Here's the drawing with two shaded views (mm, measured from the low corner). I have some questions. Round coordinates to 2 decimals unless told otherwise and drop trailing zeros. Order: outer loops, then holes, each group sorted by start corner. A loop starts at its lowest first (then second) coordinate and runs counter-clockwise, first axis right, second up. Notation, with made-up numbers: (46, 14) -> (54, 14) arc R22 cw to (54, 42) -> close; hole circle Ø2 at (18.5, 48.25). An arc over 180 degrees is marked (long way). Answer in a Markdown table with one row per item.
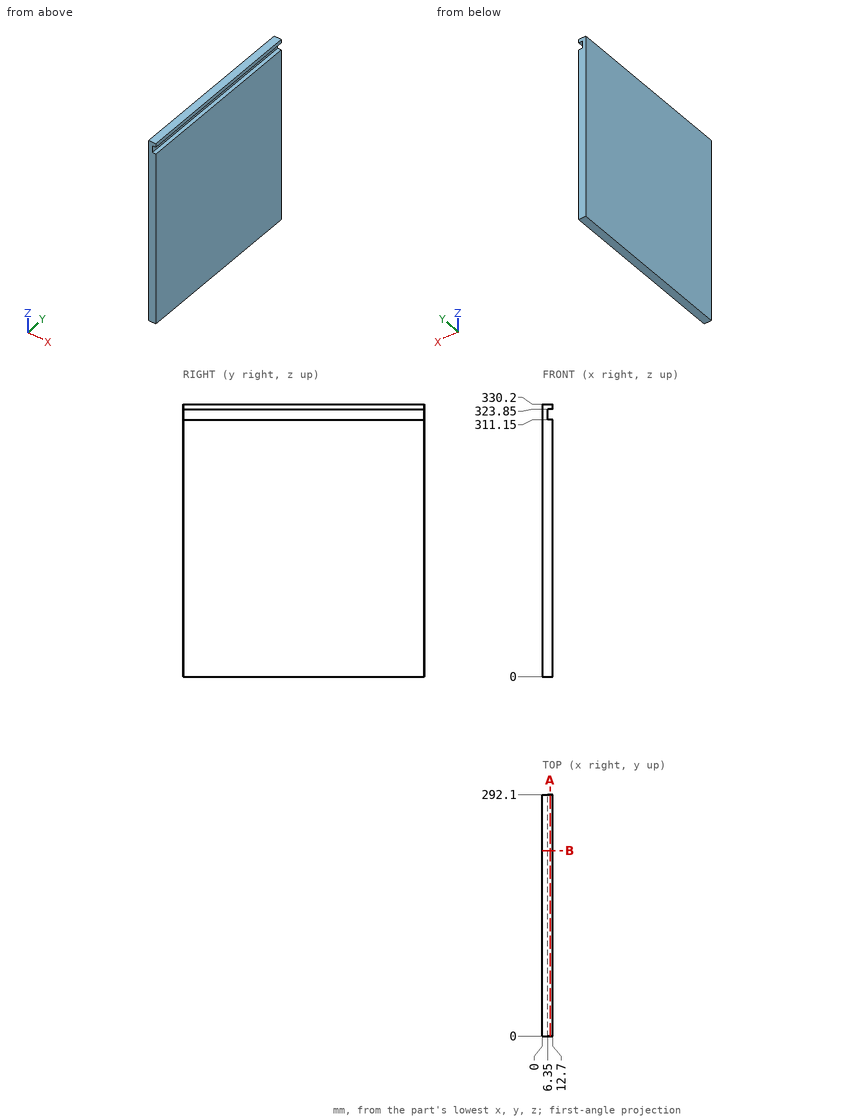
1. Please list where these lines run through material, in increasing order: line 1 along Z through (x, y) = (9.5, 264); line 2 along X through (y, z) = (162, 313).
Numbers:
| item | result |
|---|---|
| line 1 | z = 0 to 311.15, 323.85 to 330.2 |
| line 2 | x = 0 to 6.35 |
2. Suppose I cut it at B-B on y = 224.5. Write out the boundary of the cut face in (x, z).
Numbers:
| item | result |
|---|---|
| outline | (0, 0) -> (12.7, 0) -> (12.7, 311.15) -> (6.35, 311.15) -> (6.35, 323.85) -> (12.7, 323.85) -> (12.7, 330.2) -> (0, 330.2) -> close |
3. Suppose I cut it at A-A on x = 9.25. Write out the boundary of the cut face in (y, z), then the cut area to 3 significant figures.
Numbers:
| item | result |
|---|---|
| outline | (0, 0) -> (292.1, 0) -> (292.1, 311.15) -> (0, 311.15) -> close; (0, 323.85) -> (292.1, 323.85) -> (292.1, 330.2) -> (0, 330.2) -> close |
| area | 92,700 mm2 |
4. For pin 1 Ø6.5 at (y, z) = (123.5, 317) entering from +X, with a flat end and sliding along its axis, tell me the tip position at first contact or that it passes through.
Numbers:
| item | result |
|---|---|
| pin 1 | stops at x = 6.35 |
